Autodesk Inventor part; units mm, degrees
ref_plane "Start Plane" through (0, 0, 12.7) normal (0, 0, 1) x (1, 0, 0)
ref_plane "End Plane" through (0, 0, 239.3353) normal (0, 0, 1) x (1, 0, 0)
ref_plane "Work Plane5" through (19.05, 56.4661, 199.4022) normal (0, 0.5, 0.866) x (1, 0, 0)
ref_plane "Start Plane" through (0, 0, 12.7) normal (0, 0, 1) x (1, 0, 0)
ref_plane "End Plane" through (0, 0, 239.3353) normal (0, 0, 1) x (1, 0, 0)
sketch "Sketch" plane through (0, 0, 0) normal (0, 0, 1) x (1, 0, 0)
  line L0 (-12.7, 12.7) -> (12.7, 12.7)
  line L1 (12.7, 12.7) -> (12.7, -12.7)
  line L2 (12.7, -12.7) -> (-12.7, -12.7)
  line L3 (-12.7, -12.7) -> (-12.7, 12.7)
  line L4 (9.525, 9.525) -> (-9.525, 9.525)
  line L5 (-9.525, 9.525) -> (-9.525, -9.525)
  line L6 (-9.525, -9.525) -> (9.525, -9.525)
  line L7 (9.525, -9.525) -> (9.525, 9.525)
  point P0 (0, 0)
  point P1 (0, 12.7)
  point P2 (-12.7, 0)
  dimension "width" = 25.4
  dimension "d1" = 3.175
extrude "Body" add sketch "Sketch" along normal up to surface (226.6353 mm away) from surface at 12.7
sketch "Sketch4" plane through (0, 0, 0) normal (0, 0, 1) x (1, 0, 0)
  line L0 (0, 0) -> (10, 0)
ref_plane "Work Plane4" through (0, 0, 0) normal (0, -1, 0) x (1, 0, 0)
sketch "Sketch5" plane through (0, 0, 0) normal (0, -1, 0) x (1, 0, 0)
  line L0 (-2, 12.7) -> (12, 12.7)
  line L1 (-2, 239.3353) -> (12, 239.3353)
  dimension "d9" = 226.6353
ref_plane "Work Plane5" through (19.05, 56.4661, 199.4022) normal (0, 0.5, 0.866) x (1, 0, 0)
split "Split1" plane through (19.05, 56.4661, 199.4022) removes the side toward (0, 0.5, 0.866)
ref_plane "Work Plane6" through (0, 12.7, 12.7) normal (0, 0, -1) x (-1, 0, 0)
split "Split2" plane through (0, 12.7, 12.7) removes the side toward (0, 0, -1)
equation "\"G_OFFSET_START\" = -12.7"
equation "\"G_OFFSET_END\" = -14.6647"
equation "\"d4\" = -G_OFFSET_START"
equation "\"d5\" = length + G_OFFSET_END"
equation "\"G_L\" = 254"
properties part number "Square Tube Profile" material "Aluminum-6061"
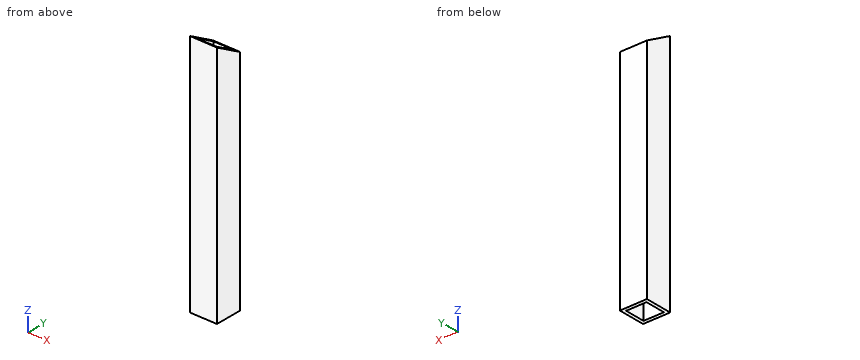
Could you check a few things on this model? Use its own coordinates, in mm. Round coordinates to 2 decimals unless told otherwise and drop trailing zeros. Order: outer loops, then holes, each group sorted by start corner. A loop starts at its lowest first (then second) coordinate and runs counter-clockwise, first axis right, second up. Notation, with made-up numbers: (-12.5, -12) -> (18.5, -12) arc R18 ccw to (18.5, 3) -> close; hole circle Ø4 at (-35.75, -24.75). An arc over 180 degrees is marked (long way). One line per question, with ' | ' between items.
Q1. If we section it at B-B on y = -7.25: Write out the boundary of the cut face in (x, z) (3 decimals).
Computed values:
outline: (-12.7, 12.7) -> (-9.525, 12.7) -> (-9.525, 236.189) -> (-12.7, 236.189) -> close; (9.525, 12.7) -> (12.7, 12.7) -> (12.7, 236.189) -> (9.525, 236.189) -> close
Q2. If I drill on line 1 (Y direction, x = 7.75, z = 31) (3 decimals); line 2 (Z direction, x = -11, y = 0.75), over which ranges is the centre line in solid material (lowest first)? Write a range as from..to.
Computed values:
line 1: -12.7..-9.525, 9.525..12.7 | line 2: 12.7..231.57
Q3. If we section it at A-A on x = -5.75: Write out the boundary of the cut face in (y, z) (3 decimals).
Computed values:
outline: (-12.7, 12.7) -> (-9.525, 12.7) -> (-9.525, 237.502) -> (-12.7, 239.335) -> close; (9.525, 12.7) -> (12.7, 12.7) -> (12.7, 224.671) -> (9.525, 226.504) -> close
Q4. If we section it at C-C on z = 142.5: Write out the boundary of the cut face in (x, y) (3 decimals).
Computed values:
outline: (-12.7, -12.7) -> (12.7, -12.7) -> (12.7, 12.7) -> (-12.7, 12.7) -> close; hole (-9.525, -9.525) -> (9.525, -9.525) -> (9.525, 9.525) -> (-9.525, 9.525) -> close
Q5. I'm going to push a flat-ended pin straight in: pin 1 (2 mm diameter, centred on x = -1.5, y = 9.5, fed in from -Z). Where does the tip first touch, or does it pass through?
Computed values:
pin 1: z = 12.7
